The model under review builds one solid part; all positions refer to its coordinate system, in mm. Round coordinates to 2 decimals unless told otherwise and drop trailing zeros. Order: outer loops, then holes, each group sorted by start corner. A loop starts at its lowest first (then second) coordinate and runs counter-clockwise, first axis right, second up.
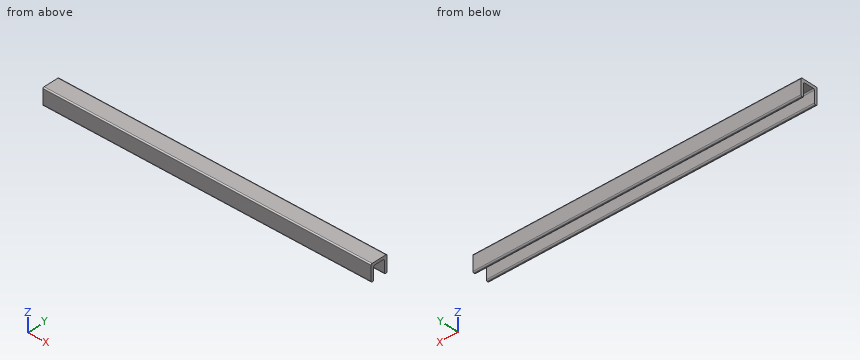
from build123d import *

# Parameters (mm, degrees)
BOSS_EXTRUDE1_START = 30
BOSS_EXTRUDE1_DEPTH = 572
CUT_EXTRUDE1_DEPTH  = 4.5


with BuildPart() as part:
    # Sketch1 → Boss-Extrude1 (new body)
    with BuildSketch(Plane(origin=(0, 0, 0), x_dir=(0, 0, -1), z_dir=(1, 0, 0)).offset(BOSS_EXTRUDE1_START)):
        with BuildLine():
            Line((-168, 10), (-188, 10))
            ThreePointArc((-188, 10), (-189.414213562, 9.414213562), (-190, 8))
            Line((-190, 8), (-190, -8))
            ThreePointArc((-190, -8), (-189.414213562, -9.414213562), (-188, -10))
            Line((-188, -10), (-168, -10))
            ThreePointArc((-168, -10), (-166.585786438, -10.585786438), (-166, -12))
            Line((-166, -12), (-166, -13))
            ThreePointArc((-166, -13), (-166.585786438, -14.414213562), (-168, -15))
            Line((-168, -15), (-193, -15))
            ThreePointArc((-193, -15), (-194.414213562, -14.414213562), (-195, -13))
            Line((-195, -13), (-195, 13))
            ThreePointArc((-195, 13), (-194.414213562, 14.414213562), (-193, 15))
            Line((-193, 15), (-168, 15))
            ThreePointArc((-168, 15), (-166.585786438, 14.414213562), (-166, 13))
            Line((-166, 13), (-166, 12))
            ThreePointArc((-166, 12), (-166.585786438, 10.585786438), (-168, 10))
        make_face()
    extrude(amount=BOSS_EXTRUDE1_DEPTH)

    # Sketch2 → Cut-Extrude1 (cut)
    with BuildSketch(Plane(origin=(0, 0, 190), x_dir=(-1, 0, 0), z_dir=(0, 0, -1))):
        with BuildLine():
            ThreePointArc((-67.75, 0), (-68.409009742, 1.590990258), (-70, 2.25))
            Line((-70, 2.25), (-560, 2.25))
            ThreePointArc((-560, 2.25), (-561.590990258, 1.590990258), (-562.25, 0))
            Line((-562.25, 0), (-67.75, 0))
        make_face()
        with BuildLine():
            ThreePointArc((-70, -2.25), (-68.409009742, -1.590990258), (-67.75, 0))
            Line((-67.75, 0), (-562.25, 0))
            ThreePointArc((-562.25, 0), (-561.590990258, -1.590990258), (-560, -2.25))
            Line((-560, -2.25), (-70, -2.25))
        make_face()
    extrude(amount=-CUT_EXTRUDE1_DEPTH, mode=Mode.SUBTRACT)


solid = part.part
(1) Clearance check with flat-ended pins moving along their axes: P1, Ø1.3, axis at x = 387.5, y = 0.5, coming from the -Z side; P2, Ø6, axis at x = 150.5, y = -0.5, coming from the -Z side; P3, Ø8, axis at y = 9, z = 179, coming from the -X side. State where each tip first meets the part, or that it passes through.
(2) We need section B-B (x = 434.5). Give the boundary of the cut face in (y, z).
(3) We need section A-A (z = 179). Give the boundary of the cut face in (x, y).
(4) To check wall thickness, follow L1, parallel to Y at x = 388, z = 168.25; L2, parallel to Y at x = 424.5, z = 167.5; L3, parallel to Z at x = 240.5, y = -2.5. State the ranges of each line that lie inside material, in increasing order.
Verdict:
1. P1: stops at z = 194.5
1. P2: stops at z = 190
1. P3: stops at x = 30
2. outline: (-15, 168) arc R2 ccw to (-13, 166) - (-12, 166) arc R2 ccw to (-10, 168) - (-10, 188) arc R2 cw to (-8, 190) - (-2.25, 190) - (-2.25, 194.5) - (2.25, 194.5) - (2.25, 190) - (8, 190) arc R2 cw to (10, 188) - (10, 168) arc R2 ccw to (12, 166) - (13, 166) arc R2 ccw to (15, 168) - (15, 193) arc R2 ccw to (13, 195) - (-13, 195) arc R2 ccw to (-15, 193) - close
3. outline: (30, -15) - (602, -15) - (602, -10) - (30, -10) - close; (30, 10) - (602, 10) - (602, 15) - (30, 15) - close
4. L1: y = -15 to -10, 10 to 15
4. L2: y = -14.94 to -10.06, 10.06 to 14.94
4. L3: z = 190 to 195
